Geometry: final body of the model. Coordinates: model frame, mm. A direction names the side the tool comes from. Coordinates: 2 decimals unless noted, no trailing zeros. Order: outer loops, then holes, each group sorted by start corner. A loop starts at its lowest first (then second) coordinate and runs counter-clockwise, first axis right, second up. Notation, with made-up numbers: (34, -1) -> (78, -1) arc R16 cw to (78, 15) -> close; hole circle Ø10 at (60, 72.5). An arc over 180 degrees is marked (long way). Answer in a Markdown table with one row per item. Add a question column.
1) Set-up query: faces 1 (the face through (-116, -3.038, -5)), 2 (the face through (495.175, -205, 60)), 3 (the face through (116.129, -1.498, 93.482)), 4 (the face through (7, -148, 147.962)). Return all of +Z, -Z, +X, -X, +Y, -Y with unobstructed straight access to the full face (end or side cutting, diameter ignored); none if empty.
2) Section query B-B on y = -89. Return the cut outline in (x, z) (3 decimals).
3) Ray query, line 1 (X direction, y = -189, z = 131.5) (3 decimals); line 2 (Y direction, x = -136, z = -117.5); line 3 (Z direction, x = -435, y = -37). Return the intervals inside material, ascending. Write a range as from..to.
4) Pull-direction query (X, two-part tool) for faces 5 (the face through (-116, 0, -5)), 6 (the face through (-281.504, -1.498, -83.885)), 7 (the face through (-495.175, -148, 60)); classes: +X half, -X half, draft (parallel to the pull), parting line (faces both ways), or undercut.
5) Section query A-A on x = 156.5. Return the cut outline in (y, z) (3 decimals).
6) Section query C-C on x = -247. Return the cut outline in (y, z) (3 decimals).
7) Contact query for flat-ended pins moving along their axis: P1, Ø5, axis at y = -2.5, z = 34, coming from the -X side; P2, Ø2.5, axis at y = -203, z = 149.5, coming from the +X side; P3, Ø2.5, axis at y = -2.5, z = 2.5, coming from the +X side; P4, Ø1, axis at x = 201, z = -103.5, coming from the +Y side. Output: stop coordinate, or through.
8) Section query D-D on y = -262.5. Return the cut outline in (x, z) (3 decimals).
```python
from build123d import *

# Parameters (mm, degrees)
BASE_FLANGE1_DEPTH           = 3.03784
EDGE_FLANGE1_STRIP_W         = 18.50136
EDGE_FLANGE1_STRIP_H         = 3.03784
EDGE_FLANGE1_STRIP_CUT_DEPTH = 984
EDGE_FLANGE1_DEPTH           = 984
EDGE_FLANGE2_DEPTH           = 278.78716
EDGE_FLANGE2_BEND_DEPTH      = 156.962160064
CUT_EXTRUDE1_DEPTH           = 594.499817979
CUT_EXTRUDE2_DEPTH           = 594.499817979
M6_START                     = -3.03784
M6_CLEARANCE_SLOT1_DEPTH     = 3.03784
M6_START_2                   = 147.96216
M6_CLEARANCE_SLOT2_DEPTH     = 3.03784


# Read off the part's stored shape, not the designer's step: M6 Clearance Slot1, M6 Clearance Slot2
# Sheet-metal steps are written as plain solids
with BuildPart() as part:
    # Sketch1 → Base-Flange1 (new body)
    with BuildSketch(Plane(origin=(0, 0, 0), x_dir=(1, 0, 0), z_dir=(0, 1, 0))):
        Polygon((334, 151), (-334, 151), (-334, 22), (-492, 22), (-492, -151), (334, -151), (492, -151), (492, 22), (334, 22), align=None)
    extrude(amount=-BASE_FLANGE1_DEPTH)

    # Edge-Flange1 strip (across the edge) → Edge-Flange1 strip cut (cut)
    with BuildSketch(Plane(origin=(492, -3.03784, 151), x_dir=(0, 0, -1), z_dir=(-1, 0, 0))):
        with Locations((-3.03784, -1.51892)):
            Rectangle(EDGE_FLANGE1_STRIP_W, EDGE_FLANGE1_STRIP_H)
    extrude(amount=EDGE_FLANGE1_STRIP_CUT_DEPTH, mode=Mode.SUBTRACT)

    # Edge-Flange1 section (across the edge) → Edge-Flange1 (add)
    with BuildSketch(Plane(origin=(492, -3.03784, 151), x_dir=(0, 0, -1), z_dir=(-1, 0, 0))):
        with BuildLine():
            Line((0, 3.175), (0, 281.96216))
            Line((0, 281.96216), (3.03784, 281.96216))
            Line((3.03784, 281.96216), (3.03784, 3.175))
            ThreePointArc((3.03784, 3.175), (3.96777597, 0.92993597), (6.21284, 0))
            Line((6.21284, 0), (6.21284, -3.03784))
            ThreePointArc((6.21284, -3.03784), (1.819698706, -1.218141294), (0, 3.175))
        make_face()
    extrude(amount=EDGE_FLANGE1_DEPTH)

    # Edge-Flange2 section (across the edge) → Edge-Flange2 (add)
    with BuildSketch(Plane(origin=(-495.175, -285, 147.96216), x_dir=(1, 0, 0), z_dir=(0, 1, 0))):
        with BuildLine():
            Line((-3.03784, 3.175), (-3.03784, 169.96216))
            Line((-3.03784, 169.96216), (0, 169.96216))
            Line((0, 169.96216), (0, 3.175))
            ThreePointArc((0, 3.175), (0.92993597, 0.92993597), (3.175, 0))
            Line((3.175, 0), (3.175, -3.03784))
            ThreePointArc((3.175, -3.03784), (-1.218141294, -1.218141294), (-3.03784, 3.175))
        make_face()
    extrude(amount=EDGE_FLANGE2_DEPTH)

    # Edge-Flange2 section 2 (across the edge) → Edge-Flange2 bend (add)
    with BuildSketch(Plane(origin=(495.175, -128.037839936, 147.96216), x_dir=(-1, 0, 0), z_dir=(0, -1, 0))):
        with BuildLine():
            Line((-3.03784, 3.175), (-3.03784, 169.96216))
            Line((-3.03784, 169.96216), (0, 169.96216))
            Line((0, 169.96216), (0, 3.175))
            ThreePointArc((0, 3.175), (0.92993597, 0.92993597), (3.175, 0))
            Line((3.175, 0), (3.175, -3.03784))
            ThreePointArc((3.175, -3.03784), (-1.218141294, -1.218141294), (-3.03784, 3.175))
        make_face()
    extrude(amount=EDGE_FLANGE2_BEND_DEPTH)

    # Sketch15 → Cut-Extrude1 (cut, through all)
    with BuildSketch(Plane(origin=(0, 0, 0), x_dir=(1, 0, 0), z_dir=(0, 1, 0))):
        with BuildLine():
            Line((492, 100.999999924), (134, 100.999999924))
            ThreePointArc((134, 100.999999924), (116.32233047, 93.677669454), (109, 75.999999924))
            Line((109, 75.999999924), (109, -76))
            ThreePointArc((109, -76), (116.32233047, -93.67766953), (134, -101))
            Line((134, -101), (492, -101))
            Line((492, -101), (492, 100.999999924))
        make_face()
    extrude(amount=-CUT_EXTRUDE1_DEPTH, mode=Mode.SUBTRACT)

    # Sketch16 → Cut-Extrude2 (cut, through all)
    with BuildSketch(Plane(origin=(0, 0, 0), x_dir=(1, 0, 0), z_dir=(0, 1, 0))):
        with BuildLine():
            Line((-334, 101), (-299, 101))
            ThreePointArc((-299, 101), (-281.5, 83.5), (-299, 66))
            Line((-299, 66), (-334, 66))
            Line((-334, 66), (-334, 101))
        make_face()
    extrude(amount=-CUT_EXTRUDE2_DEPTH, mode=Mode.SUBTRACT)

    # M6 Clearance Slot1 outline → M6 Clearance Slot1 (cut)
    with BuildSketch(Plane(origin=(0, 0, 0), x_dir=(1, 0, 0), z_dir=(0, 1, 0)).offset(M6_START)):
        with BuildLine():
            Line((319.25, 125.287839814), (319.25, 132.787839814))
            ThreePointArc((319.25, 132.787839814), (315, 137.037839814), (310.75, 132.787839814))
            Line((310.75, 132.787839814), (310.75, 125.287839814))
            ThreePointArc((310.75, 125.287839814), (315, 121.037839814), (319.25, 125.287839814))
        make_face()
        with BuildLine():
            ThreePointArc((319.25, -131.212160186), (315, -126.962160186), (310.75, -131.212160186))
            Line((310.75, -131.212160186), (310.75, -138.712160186))
            ThreePointArc((310.75, -138.712160186), (315, -142.962160186), (319.25, -138.712160186))
            Line((319.25, -138.712160186), (319.25, -131.212160186))
        make_face()
        with BuildLine():
            ThreePointArc((-310.75, -131.212160186), (-315, -126.962160186), (-319.25, -131.212160186))
            Line((-319.25, -131.212160186), (-319.25, -138.712160186))
            ThreePointArc((-319.25, -138.712160186), (-315, -142.962160186), (-310.75, -138.712160186))
            Line((-310.75, -138.712160186), (-310.75, -131.212160186))
        make_face()
        with BuildLine():
            ThreePointArc((-310.75, 132.787839814), (-315, 137.037839814), (-319.25, 132.787839814))
            Line((-319.25, 132.787839814), (-319.25, 125.287839814))
            ThreePointArc((-319.25, 125.287839814), (-315, 121.037839814), (-310.75, 125.287839814))
            Line((-310.75, 125.287839814), (-310.75, 132.787839814))
        make_face()
    extrude(amount=M6_CLEARANCE_SLOT1_DEPTH, mode=Mode.SUBTRACT)

    # M6 Clearance Slot2 outline → M6 Clearance Slot2 (cut)
    with BuildSketch(Plane.XY.offset(M6_START_2)):
        with BuildLine():
            ThreePointArc((319.250000047, -197.28784), (315.000000047, -193.03784), (310.750000047, -197.28784))
            Line((310.750000047, -197.28784), (310.750000047, -204.78784))
            ThreePointArc((310.750000047, -204.78784), (315.000000047, -209.03784), (319.250000047, -204.78784))
            Line((319.250000047, -204.78784), (319.250000047, -197.28784))
        make_face()
        with BuildLine():
            ThreePointArc((-310.750000047, -197.28784), (-315.000000047, -193.03784), (-319.250000047, -197.28784))
            Line((-319.250000047, -197.28784), (-319.250000047, -204.78784))
            ThreePointArc((-319.250000047, -204.78784), (-315.000000047, -209.03784), (-310.750000047, -204.78784))
            Line((-310.750000047, -204.78784), (-310.750000047, -197.28784))
        make_face()
    extrude(amount=M6_CLEARANCE_SLOT2_DEPTH, mode=Mode.SUBTRACT)


solid = part.part
```
Result:
| question | item | result |
|---|---|---|
| 1 | face 1 | -Z, +X, -X, -Y |
| 1 | face 2 | -Z, +Y, -Y |
| 1 | face 3 | +X, +Y, -Y |
| 1 | face 4 | -Z, -Y |
| 2 | outline | (-498.213, -22) -> (-495.175, -22) -> (-495.175, 144.787) arc R3.175 cw to (-492, 147.962) -> (492, 147.962) -> (492, 151) -> (-492, 151) arc R6.213 ccw to (-498.213, 144.787) -> close |
| 3 | line 1 | -498.213..-495.175, 495.175..498.213 |
| 3 | line 2 | -3.04..0 |
| 3 | line 3 | 147.96..151 |
| 4 | face 5 | draft |
| 4 | face 6 | -X half |
| 4 | face 7 | undercut |
| 5 | outline | (-285, 147.962) -> (-6.213, 147.962) arc R3.175 cw to (-3.038, 144.787) -> (-3.038, 101) -> (0, 101) -> (0, 144.787) arc R6.213 ccw to (-6.213, 151) -> (-285, 151) -> close; (-3.038, -151) -> (0, -151) -> (0, -101) -> (-3.038, -101) -> close |
| 6 | outline | (-285, 147.962) -> (-6.213, 147.962) arc R3.175 cw to (-3.038, 144.787) -> (-3.038, -151) -> (0, -151) -> (0, 144.787) arc R6.213 ccw to (-6.213, 151) -> (-285, 151) -> close |
| 7 | P1 | x = -492 |
| 7 | P2 | x = 497.16 |
| 7 | P3 | x = 109 |
| 7 | P4 | y = 0 |
| 8 | outline | (-498.213, -22) -> (-495.175, -22) -> (-495.175, 144.787) arc R3.175 cw to (-492, 147.962) -> (492, 147.962) arc R3.175 cw to (495.175, 144.787) -> (495.175, -22) -> (498.213, -22) -> (498.213, 144.787) arc R6.213 ccw to (492, 151) -> (-492, 151) arc R6.213 ccw to (-498.213, 144.787) -> close |
